```python
from build123d import *

# Parameters (mm, degrees)
SKETCH1_R               = 50.8
TOP_PLATE_DEPTH         = 11.938
SKETCH2_R               = 6.35
CENTRAL_HOLE_DEPTH      = 73.82716419
SKETCH3_R               = 4.66627796
BALL_HOLE_DEPTH         = 11.938
BALL_HOLE_PATTERN_COUNT = 3


with BuildPart() as part:
    # Sketch1 → top_plate (new body)
    with BuildSketch(Plane.XY):
        Circle(SKETCH1_R)
    extrude(amount=TOP_PLATE_DEPTH)

    # Sketch2 → central_hole (cut, through all)
    with BuildSketch(Plane.XY.offset(11.938)):
        Circle(SKETCH2_R)
    extrude(amount=-CENTRAL_HOLE_DEPTH, mode=Mode.SUBTRACT)

    # Sketch3 → ball_hole (cut)
    with BuildSketch(Plane.XY.offset(11.938)):
        with Locations((0, 31.75)):
            Circle(SKETCH3_R)
    ball_hole = extrude(amount=-BALL_HOLE_DEPTH, mode=Mode.SUBTRACT)

    # ball_hole_pattern: ball_hole ×3 about axis
    ball_hole_pattern_axis = Axis((0, 0, 0), (0, 0, 1))
    for i in range(1, BALL_HOLE_PATTERN_COUNT):
        add(ball_hole.rotate(ball_hole_pattern_axis, i * 360 / BALL_HOLE_PATTERN_COUNT), mode=Mode.SUBTRACT)


solid = part.part
```
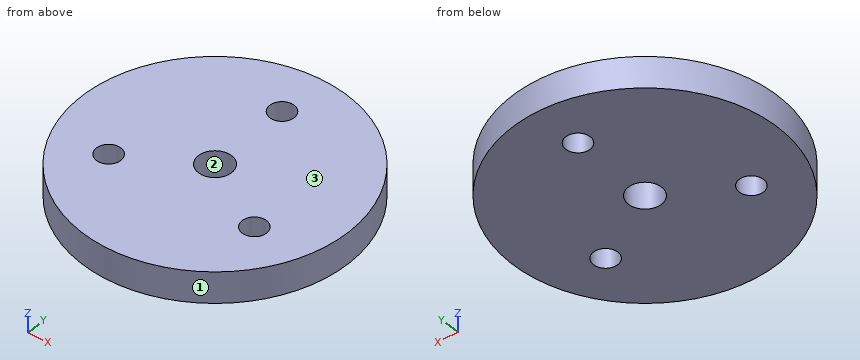
Geometry check sheet. Reference: the model listing, model coordinates, mm. Face numbers are marked on the shaded views. Give positions to 0.01 mm unless a question says otherwise; leave off trailing zeros. Write each loop counter-clockwise with the first axis right and the second up, starting at its lowest first coordinate (ties: lowest second). Pieces come first, ordered by that corner, then holes. Notation, with made-up numbers: (57, -18) -> (76, -18) arc R21 cw to (76, -8) -> close; hole circle Ø10 at (25, -16). An arc over 180 degrees is marked (long way). Use one line per item in the form item = value.
Item 1: Sectioned sample at D-D on z = 6.5. Enter the section's corners in (x, y) (3 decimals).
Results list:
outline = circle Ø101.6 at (0, 0); hole circle Ø9.333 at (-27.496, -15.875); hole circle Ø12.7 at (0, 0); hole circle Ø9.333 at (0, 31.75); hole circle Ø9.333 at (27.496, -15.875)
Item 2: Depth check by flat-ended pin: pin 1 Ø2 at (y, z) = (10.5, 4) entering from -X; pin 2 Ø1.5 at (x, z) = (25.5, 8) entering from -Y; pin 3 Ø8.5 at (x, y) = (27.5, -15.88) entering from -Z; pin 4 Ø1 at (x, z) = (1, 4.5) entering from -Y. Enter the tip coordinate at first touch or a pass-through.
Results list:
pin_1 = -49.9
pin_2 = -44.36
pin_3 = through
pin_4 = -50.8
Item 3: Sectioned sample at C-C on x = -27. Enter the section's corners in (y, z).
Results list:
outline = (-43.03, 0) -> (-20.51, 0) -> (-20.51, 11.94) -> (-43.03, 11.94) -> close; (-11.24, 0) -> (43.03, 0) -> (43.03, 11.94) -> (-11.24, 11.94) -> close
Item 4: Mould release check, pull along Y, two halves, no side actions. Record for the marked faces 1, 2 and 3: released by +Y, released by -Y, zero draft, split by the parting line, or undercut.
Results list:
face_1 = split by the parting line
face_2 = undercut
face_3 = zero draft
Item 5: Sectioned sample at A-A on x = 0. Enter the section's corners in (y, z).
Results list:
outline = (-50.8, 0) -> (-6.35, 0) -> (-6.35, 11.94) -> (-50.8, 11.94) -> close; (6.35, 0) -> (27.08, 0) -> (27.08, 11.94) -> (6.35, 11.94) -> close; (36.42, 0) -> (50.8, 0) -> (50.8, 11.94) -> (36.42, 11.94) -> close
Item 6: Sectioned sample at B-B on y = 0. Enter the section's corners in (x, z), plus the area to 3 significant figures.
Results list:
outline = (-50.8, 0) -> (-6.35, 0) -> (-6.35, 11.94) -> (-50.8, 11.94) -> close; (6.35, 0) -> (50.8, 0) -> (50.8, 11.94) -> (6.35, 11.94) -> close
area = 1,060 mm2
Item 7: Scan lines: line 1 (Y direction, x = 0, z = 8.5); line 2 (Y direction, x = -3.5, z = 5.25); line 3 (X direction, y = -16, z = 3.75). Record each from-to range of solid material in increasing order.
Results list:
line_1 = -50.8 to -6.35, 6.35 to 27.08, 36.42 to 50.8
line_2 = -50.68 to -5.3, 5.3 to 28.66, 34.84 to 50.68
line_3 = -48.21 to -32.16, -22.83 to 22.83, 32.16 to 48.21
